```python
from build123d import *

# Parameters (mm, degrees)
SKETCH3_W                = 6.5
SKETCH3_H                = 6.5
BOSS_EXTRUDE1_DEPTH      = 200
BOSS_EXTRUDE1_2_DEPTH    = 200
BOSS_EXTRUDE1_3_DEPTH    = 200
BOSS_EXTRUDE1_4_DEPTH    = 200
SKETCH11_W               = 100
SKETCH11_H               = 100
SKETCH11_W_2             = 87
SKETCH11_H_2             = 87
BOSS_EXTRUDE7_DEPTH      = 6.5
BOSS_EXTRUDE8_DEPTH      = 3.25
BOSS_EXTRUDE8_DEPTH_BACK = 3.25
BOSS_EXTRUDE8_START      = -100
SKETCH12_W               = 100
SKETCH12_H               = 100
SKETCH12_W_2             = 87
SKETCH12_H_2             = 87
SKETCH13_W               = 6.5
SKETCH13_H               = 6.5
BOSS_EXTRUDE9_DEPTH      = 13.5
SKETCH14_W               = 6.5
SKETCH14_H               = 6.5
BOSS_EXTRUDE10_DEPTH     = 13.5


with BuildPart() as part:
    # Sketch3 → Boss-Extrude1 (new body)
    with BuildSketch(Plane(origin=(0, 0, 0), x_dir=(1, 0, 0), z_dir=(0, 1, 0))):
        with Locations((-46.75, 46.75)):
            Rectangle(SKETCH3_W, SKETCH3_H)
    extrude(amount=BOSS_EXTRUDE1_DEPTH)



with BuildPart() as body_2:
    # Sketch3 → Boss-Extrude1 2 (new body)
    with BuildSketch(Plane(origin=(0, 0, 0), x_dir=(1, 0, 0), z_dir=(0, 1, 0))):
        with Locations((46.75, 46.75)):
            Rectangle(SKETCH3_W, SKETCH3_H)
    extrude(amount=BOSS_EXTRUDE1_2_DEPTH)


with BuildPart() as body_3:
    # Sketch3 → Boss-Extrude1 3 (new body)
    with BuildSketch(Plane(origin=(0, 0, 0), x_dir=(1, 0, 0), z_dir=(0, 1, 0))):
        with Locations((46.75, -46.75)):
            Rectangle(SKETCH3_W, SKETCH3_H)
    extrude(amount=BOSS_EXTRUDE1_3_DEPTH)


with BuildPart() as body_4:
    # Sketch3 → Boss-Extrude1 4 (new body)
    with BuildSketch(Plane(origin=(0, 0, 0), x_dir=(1, 0, 0), z_dir=(0, 1, 0))):
        with Locations((-46.75, -46.75)):
            Rectangle(SKETCH3_W, SKETCH3_H)
    extrude(amount=BOSS_EXTRUDE1_4_DEPTH)


with BuildPart() as part_1:
    add(part.part)

    add(body_2.part)  # Boss-Extrude7 merges body 2

    add(body_3.part)  # Boss-Extrude7 merges body 3

    add(body_4.part)  # Boss-Extrude7 merges body 4
    # Sketch11 → Boss-Extrude7 (add)
    with BuildSketch(Plane(origin=(0, 200, 0), x_dir=(1, 0, 0), z_dir=(0, 1, 0))):
        Rectangle(SKETCH11_W, SKETCH11_H)
        Rectangle(SKETCH11_W_2, SKETCH11_H_2, mode=Mode.SUBTRACT)
    extrude(amount=-BOSS_EXTRUDE7_DEPTH)

    # Sketch12 → Boss-Extrude8 (add, two sides: drawn at the far end of the back side and taken through both)
    with BuildSketch(Plane(origin=(0, 200, 0), x_dir=(1, 0, 0), z_dir=(0, 1, 0)).offset(BOSS_EXTRUDE8_START - BOSS_EXTRUDE8_DEPTH_BACK)):
        Rectangle(SKETCH12_W, SKETCH12_H)
        Rectangle(SKETCH12_W_2, SKETCH12_H_2, mode=Mode.SUBTRACT)
    extrude(amount=BOSS_EXTRUDE8_DEPTH + BOSS_EXTRUDE8_DEPTH_BACK)

    # Sketch13 → Boss-Extrude9 (add)
    with BuildSketch(Plane(origin=(0, 200, 0), x_dir=(1, 0, 0), z_dir=(0, 1, 0))):
        with Locations((-46.75, 46.75)):
            Rectangle(SKETCH13_W, SKETCH13_H)
        with Locations((46.75, 46.75)):
            Rectangle(SKETCH13_W, SKETCH13_H)
        with Locations((46.75, -46.75)):
            Rectangle(SKETCH13_W, SKETCH13_H)
        with Locations((-46.75, -46.75)):
            Rectangle(SKETCH13_W, SKETCH13_H)
    extrude(amount=BOSS_EXTRUDE9_DEPTH)

    # Sketch14 → Boss-Extrude10 (add)
    with BuildSketch(Plane.XZ):
        with Locations((-46.75, 46.75)):
            Rectangle(SKETCH14_W, SKETCH14_H)
        with Locations((46.75, 46.75)):
            Rectangle(SKETCH14_W, SKETCH14_H)
        with Locations((46.75, -46.75)):
            Rectangle(SKETCH14_W, SKETCH14_H)
        with Locations((-46.75, -46.75)):
            Rectangle(SKETCH14_W, SKETCH14_H)
    extrude(amount=BOSS_EXTRUDE10_DEPTH)


solid = part_1.part
```
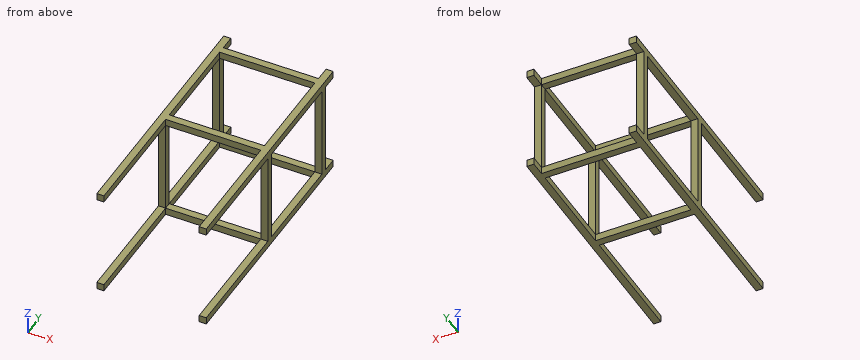
Input: part model. Units: mm. Frame: model coordinates. Give positions to 0.01 mm unless a question says otherwise; leave off trailing zeros. Order: outer loops, then holes, each group sorted by start corner. A loop starts at its lowest first (then second) coordinate and runs counter-clockwise, first axis right, second up. Notation, with made-up numbers: M 64,-18 L 96,-18 A14 ccw 96,6 Z; hole C 72,9 d11. An arc over 180 degrees is marked long. One line per question, with ' | ' between items. Start each with the question number.
1. Section query B-B (y = 110.5). Return the cut outline in (x, z), and give its area (3 significant figures).
2. Section query A-A (z = 2.5). Return the cut outline in (x, y).
3. First-contact query: pin 1 Ø3 at (x, z) = (-45, 16.5) entering from +Y; pin 2 Ø5 at (x, z) = (5.5, -46) entering from -Y; pin 3 Ø12 at (x, y) = (-39.5, 50.5) entering from -Z. Flat tips, straight axial feed; report the tip coordinate or a pass-through.
4. Material intervals for probe 1 along X at (y, z) = (195, -22), sorted ascending. Write a range as [from, to].
Here are the results:
1) outline: M -50,-50 L -43.5,-50 L -43.5,-43.5 L -50,-43.5 Z; M -50,43.5 L -43.5,43.5 L -43.5,50 L -50,50 Z; M 43.5,-50 L 50,-50 L 50,-43.5 L 43.5,-43.5 Z; M 43.5,43.5 L 50,43.5 L 50,50 L 43.5,50 Z | area: 169 mm²
2) outline: M -50,96.75 L -43.5,96.75 L -43.5,103.25 L -50,103.25 Z; M -50,193.5 L -43.5,193.5 L -43.5,200 L -50,200 Z; M 43.5,96.75 L 50,96.75 L 50,103.25 L 43.5,103.25 Z; M 43.5,193.5 L 50,193.5 L 50,200 L 43.5,200 Z
3) pin 1: y = 200 | pin 2: y = 96.75 | pin 3: z = -50
4) probe 1: [-50, -43.5], [43.5, 50]
